CAD build for the part. Positions are in the model's coordinates, mm. Give positions to 0.01 mm unless a question says otherwise; leave off trailing zeros. Answer as CSV lines item,"result".
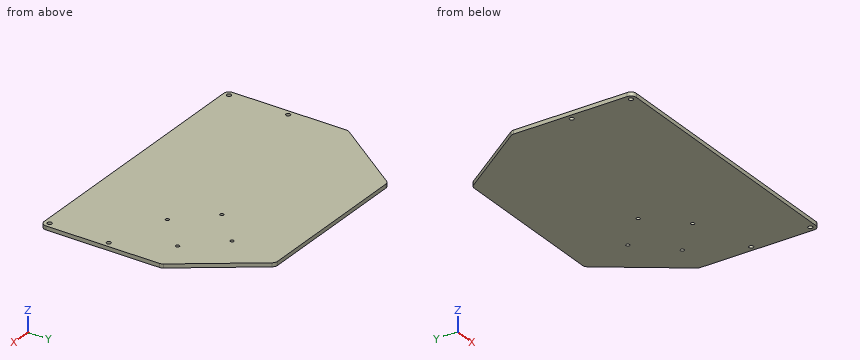
from build123d import *

# Parameters (mm, degrees)
BOSS_EXTRU_1_DEPTH           = 3.5
ESQUISSE2_R                  = 2
ENL_V_MAT_EXTRU_1_DEPTH      = 395.382111663
ENL_V_MAT_EXTRU_2_DEPTH      = 395.382111663
ENL_V_MAT_EXTRU_2_DEPTH_BACK = 395.382111663
CONG_1_R                     = 5
ESQUISSE4_R                  = 1.6
ENL_V_MAT_EXTRU_4_DEPTH      = 309.078317965


with BuildPart() as part:
    # Esquisse1 → Boss.-Extru.1 (new body)
    with BuildSketch(Plane.XY):
        with BuildLine():
            Line((5, 0), (245, 0))
            ThreePointArc((245, 0), (248.535533906, 1.464466094), (250, 5))
            Line((250, 5), (250, 305))
            Line((250, 305), (0, 305))
            Line((0, 305), (0, 5))
            ThreePointArc((0, 5), (1.464466094, 1.464466094), (5, 0))
        make_face()
    extrude(amount=BOSS_EXTRU_1_DEPTH)

    # Esquisse2 → Enlèv. mat.-Extru.1 (cut, through all)
    with BuildSketch(Plane.XY.offset(3.5)):
        with Locations((5, 5)):
            Circle(ESQUISSE2_R)
        with Locations((245, 5)):
            Circle(ESQUISSE2_R)
        with Locations((5, 58.8)):
            Circle(ESQUISSE2_R)
        with Locations((245, 58.8)):
            Circle(ESQUISSE2_R)
    extrude(amount=-ENL_V_MAT_EXTRU_1_DEPTH, mode=Mode.SUBTRACT)

    # Esquisse3 → Enlèv. mat.-Extru.2 (cut, two sides: drawn at the far end of the back side and taken through both)
    with BuildSketch(Plane.XY.offset(3.5).offset(-ENL_V_MAT_EXTRU_2_DEPTH_BACK)):
        Polygon((-374.383398967, -414.136758554), (0, 110), (50, 180), (200, 180), (250, 110), (624.383398967, -414.136758554), (624.383398967, 874.090350445), (-374.383398967, 874.090350445), align=None)
    extrude(amount=ENL_V_MAT_EXTRU_2_DEPTH + ENL_V_MAT_EXTRU_2_DEPTH_BACK, mode=Mode.SUBTRACT)

    # Congé1
    cong_1_edges = [part.edges().sort_by_distance(p)[0] for p in [
        (50, 180, 1.75),
        (200, 180, 1.75),
        (250, 110, 1.75),
        (0, 110, 1.75),
    ]]
    fillet(cong_1_edges, radius=CONG_1_R)

    # Esquisse4 → Enlèv. mat.-Extru.4 (cut, through all)
    with BuildSketch(Plane.XY.offset(3.5)):
        with Locations((220, 104.5)):
            Circle(ESQUISSE4_R)
        with Locations((190.499010186, 134)):
            Circle(ESQUISSE4_R)
        with Locations((160.998020372, 104.5)):
            Circle(ESQUISSE4_R)
        with Locations((190.499010186, 75)):
            Circle(ESQUISSE4_R)
    extrude(amount=-ENL_V_MAT_EXTRU_4_DEPTH, mode=Mode.SUBTRACT)


solid = part.part
1) Flat gauge pin, fed straight in: pin 1 (1.5 mm diameter, centred on y = 149, z = 2, fed in from +X). Where does the tip first touch, or does it go through?
Answer below:
pin 1,"stops at x = 222.68"
2) Band-saw the part on A-A on z = 1. Give the number of separate pieces and of enclosed holes in the cut face, and give its area (3 significant figures).
Answer below:
separate pieces,"1"
enclosed holes,"8"
area,"41,400 mm^2"
3) Drill centre lines: line 1 (Y direction, x = 5, z = 2.6); line 2 (X direction, y = 75.5, z = 2.1); line 3 (X direction, y = 169.5, z = 2.05). Where is each one in solid material? Low to high. Write a range as from..to.
Answer below:
line 1,"y = 0..3, 7..56.8, 60.8..117"
line 2,"x = 0..188.98, 192.02..250"
line 3,"x = 42.5..207.5"
